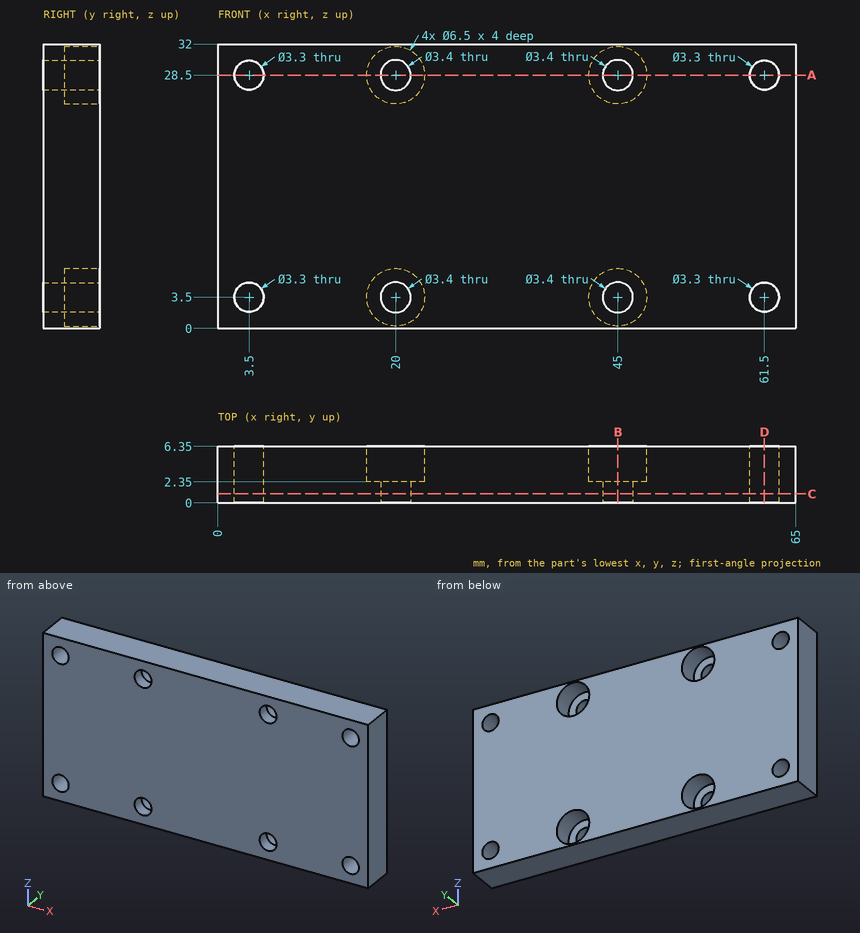
Answer from the drawing. Dimensions are ordinates in mm from the lowest x, y and z of the part. Round coordinates to 2 decimals unless told otherwise and drop trailing zeros. Write each loop counter-clockwise with the first axis right and the second up, starting at its lowest first coordinate (ties: lowest second). Pieces come first, ordered by that corner, then holes.
1. The part is cut by section A-A, the plane z = 28.5. Determine the outline of the cut face in (x, y).
2. The part is cut by section C-C, the plane y = 1. State how many separate pieces and enclosed holes the cut face has, then the cut area to 3 significant figures.
3. The part is cut by section D-D, the plane x = 61.5. Determine the outline of the cut face in (y, z), then the cut area to 3 significant figures.
4. The part is cut by section B-B, the plane x = 45. Determine the outline of the cut face in (y, z).
5. Straight lines are drawn through the part: L1, parallel to X at y = 5.75, z = 3.5; L2, parallel to X at y = 1.15, z = 3.5; L3, parallel to Z at x = 3.5, y = 4. For each, find the intervals that lie inside material, in ascending order.
6. Given pin 1 Ø3 at (y, z) = (4, 24) entering from -X; pin 2 Ø2 at (x, z) = (21, 4) entering from +Y, each flat-ended and moving along its own axis, determine where each tip first touches the part or whether it passes through.
Values:
1. outline: (0, 0) - (1.85, 0) - (1.85, 6.35) - (0, 6.35) - close; (5.15, 0) - (18.3, 0) - (18.3, 2.35) - (16.75, 2.35) - (16.75, 6.35) - (5.15, 6.35) - close; (21.7, 0) - (43.3, 0) - (43.3, 2.35) - (41.75, 2.35) - (41.75, 6.35) - (23.25, 6.35) - (23.25, 2.35) - (21.7, 2.35) - close; (46.7, 0) - (59.85, 0) - (59.85, 6.35) - (48.25, 6.35) - (48.25, 2.35) - (46.7, 2.35) - close; (63.15, 0) - (65, 0) - (65, 6.35) - (63.15, 6.35) - close
2. separate pieces: 1
2. enclosed holes: 8
2. area: 2,010 mm2
3. outline: (0, 0) - (6.35, 0) - (6.35, 1.85) - (0, 1.85) - close; (0, 5.15) - (6.35, 5.15) - (6.35, 26.85) - (0, 26.85) - close; (0, 30.15) - (6.35, 30.15) - (6.35, 32) - (0, 32) - close
3. area: 161 mm2
4. outline: (0, 0) - (6.35, 0) - (6.35, 0.25) - (2.35, 0.25) - (2.35, 1.8) - (0, 1.8) - close; (0, 5.2) - (2.35, 5.2) - (2.35, 6.75) - (6.35, 6.75) - (6.35, 25.25) - (2.35, 25.25) - (2.35, 26.8) - (0, 26.8) - close; (0, 30.2) - (2.35, 30.2) - (2.35, 31.75) - (6.35, 31.75) - (6.35, 32) - (0, 32) - close
5. L1: x = 0 to 1.85, 5.15 to 16.75, 23.25 to 41.75, 48.25 to 59.85, 63.15 to 65
5. L2: x = 0 to 1.85, 5.15 to 18.3, 21.7 to 43.3, 46.7 to 59.85, 63.15 to 65
5. L3: z = 0 to 1.85, 5.15 to 26.85, 30.15 to 32
6. pin 1: stops at x = 0
6. pin 2: stops at y = 2.35
